Autodesk Inventor part; units mm, degrees
ref_plane "YZ Plane" through (0, 0, 0) normal (1, 0, 0) x (0, 1, 0)
ref_plane "XZ Plane" through (0, 0, 0) normal (0, 1, 0) x (-1, 0, 0)
ref_plane "XY Plane" through (0, 0, 0) normal (0, 0, 1) x (1, 0, 0)
sketch "스케치1" plane through (0, 0, 0) normal (0, 0, 1) x (1, 0, 0)
  line L0 (28.124, 3.5) -> (28.124, -58.5)
  line L1 (-12.7588, 3.5) -> (-12.7588, -58.5)
  line L2 (-12.7588, -58.5) -> (28.124, -58.5)
  line L3 (-12.7588, 3.5) -> (-12.7588, 4.4)
  line L4 (28.124, 4.4) -> (28.124, 3.5)
  line L5 (-12.7588, 4.4) -> (-12.7588, 10)
  line L6 (-12.7588, 10) -> (28.124, 10)
  line L7 (28.124, 10) -> (28.124, 4.4)
  dimension "d16" = 68.5
  dimension "d50" = 40.8828
extrude "돌출2" add sketch "스케치1" along normal blind 4
sketch "스케치4" plane through (0, 0, 4) normal (0, 0, 1) x (1, 0, 0)
  circle A0 centre (7.6826, -9.5) radius 5
  point P0 (0, 0)
sketch "스케치6" plane through (0, 0, 4) normal (0, 0, 1) x (1, 0, 0)
  circle A0 centre (7.6826, -9.5) radius 13 construction
  line L0 (7.6826, -9.5) -> (-1.5098, -0.3076) construction
  line L1 (7.6826, -9.5) -> (20.6826, -9.5) construction
  line L2 (7.6826, -9.5) -> (-1.5098, -18.6924) construction
  line L3 (7.6826, -9.5) -> (20.6826, -9.5) construction
  circle A1 centre (-1.5098, -0.3076) radius 1.6
  circle A2 centre (-1.5098, -18.6924) radius 1.6
  circle A3 centre (7.6826, -9.5) radius 5
  circle A4 centre (16.875, -0.3076) radius 1.6
  line L4 (7.6826, -9.5) -> (16.875, -18.6924) construction
  circle A5 centre (16.875, -18.6924) radius 1.6
  point P0 (0, 0)
  dimension "d51" = 26
  dimension "d52" = 135
  dimension "d53" = 135
  dimension "d54" = 3.2
  dimension "d55" = 3.2
  dimension "d56" = 3.2
  dimension "d57" = 3.2
extrude "돌출4" cut sketch "스케치6" against normal up to surface (4 mm away)
sketch "스케치5" plane through (0, 0, 4) normal (0, 0, 1) x (1, 0, 0)
  line L0 (-12.7588, 10) -> (-12.7588, -58.5)
  line L1 (-12.7588, -58.5) -> (28.124, -58.5)
  line L2 (28.124, -58.5) -> (28.124, 10)
  line L3 (28.124, 10) -> (-12.7588, 10)
  circle A0 centre (-9.7588, -59.5) radius 1.6
  circle A1 centre (25.124, -59.5) radius 1.6
  circle A2 centre (-9.2588, 10.5) radius 1.6
  circle A3 centre (24.624, 10.5) radius 1.6
  line L4 (28.124, 10) -> (28.124, 14)
  line L5 (28.124, -58.5) -> (28.124, 10)
  line L6 (28.124, -58.5) -> (28.124, -62.5)
  point P0 (0, 0)
  dimension "d36" = 3.2
  dimension "d37" = 3.2
  dimension "d38" = 3.2
  dimension "d39" = 3.2
  dimension "d40" = 3
  dimension "d42" = 3.5
  dimension "d44" = 3.5
  dimension "d46" = 3
  dimension "d64" = 4
  dimension "d65" = 3.5
  dimension "d66" = 3.5
  dimension "d67" = 4
  dimension "d68" = 3
  dimension "d69" = 3
extrude "돌출3" cut sketch "스케치5" against normal up to surface (4 mm away) contours A2 L3 | L3 A2 | A0 L1 | L1 A0 | A3 L3 | L3 A3 | A1 L1 | L1 A1
sketch "스케치7" plane through (0, 0, 4) normal (0, 0, 1) x (1, 0, 0)
  line L0 (-12.7588, 10) -> (-12.7588, 14)
  arc A0 (23.1041, 10) -> (26.1439, 10) centre (24.624, 10.5) ccw
  arc A1 (26.373, -58.5) -> (23.875, -58.5) centre (25.124, -59.5) ccw
  arc A2 (-10.7787, 10) -> (-7.7389, 10) centre (-9.2588, 10.5) ccw
  arc A3 (-8.5098, -58.5) -> (-11.0078, -58.5) centre (-9.7588, -59.5) ccw
  circle A4 centre (16.875, -0.3076) radius 1.6
  circle A5 centre (-1.5098, -18.6924) radius 1.6
  circle A6 centre (7.6826, -9.5) radius 5
  circle A7 centre (16.875, -18.6924) radius 1.6
  circle A8 centre (-1.5098, -0.3076) radius 1.6
  line L1 (-12.7588, -58.5) -> (-11.0078, -58.5)
  line L2 (28.124, -58.5) -> (28.124, 10)
  line L3 (28.124, 10) -> (26.1439, 10)
  line L4 (-12.7588, 10) -> (-12.7588, -58.5)
  line L5 (28.124, 10) -> (28.124, 14)
  line L6 (28.124, 14) -> (-12.7588, 14)
  line L7 (28.124, -58.5) -> (28.124, 10)
  line L8 (-12.7588, -58.5) -> (28.124, -58.5)
  line L9 (28.124, -58.5) -> (-12.7588, -58.5)
  line L10 (-12.7588, -58.5) -> (-12.7588, -62.5)
  line L11 (-12.7588, -62.5) -> (28.124, -62.5)
  line L12 (28.124, -62.5) -> (28.124, -58.5)
  line L13 (23.1041, 10) -> (-7.7389, 10)
  line L14 (-10.7787, 10) -> (-12.7588, 10)
  line L15 (-8.5098, -58.5) -> (23.875, -58.5)
  line L16 (26.373, -58.5) -> (28.124, -58.5)
  circle A9 centre (24.624, 10.5) radius 1.6
  arc A10 (-10.7787, 10) -> (-7.7389, 10) centre (-9.2588, 10.5) ccw
  circle A11 centre (-9.2588, 10.5) radius 1.6
  circle A12 centre (25.124, -59.5) radius 1.6
  arc A13 (-8.5098, -58.5) -> (-11.0078, -58.5) centre (-9.7588, -59.5) ccw
  circle A14 centre (-9.7588, -59.5) radius 1.6
  point P0 (0, 0)
  point P1 (26.373, -58.5)
  point P2 (23.875, -58.5)
  point P3 (-7.7389, 10)
  dimension "d60" = 4
  dimension "d61" = 4
extrude "돌출6" add sketch "스케치7" against normal up to surface (4 mm away) contours L0 L6 L5 L3 A9 L13 A11 L14 | L1 A14 L8 A12 L12 L11 L10
fillet "모깎기3" radius 2 4 edges at (28.124, 14, 2) (-12.7588, 14, 2) (-12.7588, -62.5, 2) (28.124, -62.5, 2)
sketch "스케치10" plane through (0, 0, 4) normal (0, 0, 1) x (1, 0, 0)
  line L0 (-3.7588, -53.5) -> (19.124, -53.5)
  line L1 (21.124, -51.5) -> (21.124, -27.5)
  line L2 (19.124, -25.5) -> (-3.7588, -25.5)
  line L3 (-5.7588, -27.5) -> (-5.7588, -51.5)
  circle A0 centre (-9.7588, -59.5) radius 1.6
  line L4 (28.124, -60.5) -> (28.124, 12)
  line L5 (-12.7588, 12) -> (-12.7588, -60.5)
  circle A1 centre (25.124, -59.5) radius 1.6
  circle A2 centre (24.624, 10.5) radius 1.6
  circle A3 centre (-9.2588, 10.5) radius 1.6
  circle A4 centre (16.875, -0.3076) radius 1.6
  circle A5 centre (-1.5098, -18.6924) radius 1.6
  circle A6 centre (7.6826, -9.5) radius 5
  circle A7 centre (16.875, -18.6924) radius 1.6
  circle A8 centre (-1.5098, -0.3076) radius 1.6
  arc A9 (-5.7588, -51.5) -> (-3.7588, -53.5) centre (-3.7588, -51.5) ccw
  arc A10 (19.124, -53.5) -> (21.124, -51.5) centre (19.124, -51.5) ccw
  arc A11 (21.124, -27.5) -> (19.124, -25.5) centre (19.124, -27.5) ccw
  arc A12 (-3.7588, -25.5) -> (-5.7588, -27.5) centre (-3.7588, -27.5) ccw
  arc A13 (26.124, -62.5) -> (28.124, -60.5) centre (26.124, -60.5) ccw
  arc A14 (28.124, 12) -> (26.124, 14) centre (26.124, 12) ccw
  line L6 (26.124, 14) -> (-10.7588, 14)
  arc A15 (-10.7588, 14) -> (-12.7588, 12) centre (-10.7588, 12) ccw
  arc A16 (-12.7588, -60.5) -> (-10.7588, -62.5) centre (-10.7588, -60.5) ccw
  line L7 (-10.7588, -62.5) -> (26.124, -62.5)
  point P0 (0, 0)
  point P1 (-5.7588, -53.5)
  point P2 (21.124, -25.5)
  point P3 (21.124, -53.5)
  point P4 (-5.7588, -25.5)
  dimension "d84" = 16
  dimension "d87" = 7
  dimension "d88" = 7
  dimension "d89" = 2
extrude "돌출7" cut sketch "스케치10" against normal up to surface (4 mm away) contours A9 L3 A12 L2 A11 L1 A10 L0
sketch "스케치11" plane through (0, 0, 4) normal (0, 0, 1) x (1, 0, 0)
  line L0 (-10.7588, 14) -> (26.124, 14)
  line L1 (7.6826, 14) -> (7.6826, -136) construction
  circle A0 centre (7.6826, -79.433) radius 20
  arc A1 (21.124, -27.5) -> (19.124, -25.5) centre (19.124, -27.5) ccw
  line L2 (21.124, -27.5) -> (21.124, -51.5)
  arc A2 (19.124, -53.5) -> (21.124, -51.5) centre (19.124, -51.5) ccw
  line L3 (19.124, -53.5) -> (-3.7588, -53.5)
  arc A3 (-5.7588, -51.5) -> (-3.7588, -53.5) centre (-3.7588, -51.5) ccw
  line L4 (-5.7588, -51.5) -> (-5.7588, -27.5)
  arc A4 (-3.7588, -25.5) -> (-5.7588, -27.5) centre (-3.7588, -27.5) ccw
  line L5 (-3.7588, -25.5) -> (19.124, -25.5)
  circle A5 centre (25.124, -59.5) radius 1.6
  circle A6 centre (-9.7588, -59.5) radius 1.6
  line L6 (28.124, -60.5) -> (28.124, 12)
  line L7 (-12.7588, 12) -> (-12.7588, -60.5)
  circle A7 centre (24.624, 10.5) radius 1.6
  circle A8 centre (-9.2588, 10.5) radius 1.6
  circle A9 centre (16.875, -0.3076) radius 1.6
  circle A10 centre (-1.5098, -18.6924) radius 1.6
  circle A11 centre (7.6826, -9.5) radius 5
  circle A12 centre (16.875, -18.6924) radius 1.6
  circle A13 centre (-1.5098, -0.3076) radius 1.6
  arc A14 (26.124, -62.5) -> (28.124, -60.5) centre (26.124, -60.5) ccw
  arc A15 (28.124, 12) -> (26.124, 14) centre (26.124, 12) ccw
  line L8 (26.124, 14) -> (-10.7588, 14)
  arc A16 (-10.7588, 14) -> (-12.7588, 12) centre (-10.7588, 12) ccw
  arc A17 (-12.7588, -60.5) -> (-10.7588, -62.5) centre (-10.7588, -60.5) ccw
  line L9 (-10.7588, -62.5) -> (26.124, -62.5)
  point P0 (0, 0)
  point P1 (-2.9604, -62.5)
  point P2 (18.3256, -62.5)
  dimension "d90" = 150
  dimension "d91" = 40
  dimension "d92" = 25.933
extrude "돌출8" cut sketch "스케치11" against normal up to surface (4 mm away) contours A0 L9 picked at (6.936, -61.5196)
properties part number "링크2고정부" material "알루미늄 6061"
The listing builds one solid part. Answer for the finished solid, in the listing's coordinates (mm). A direction names the side the tool comes from. Round coordinates to 2 decimals unless told otherwise and drop trailing zeros. Loops run counter-clockwise (first coordinate to the right, second up) from the corner with the lowest first, then second, coordinate; pieces in that order, holes last.
Q1. Which of the six approach directions +Z, -Z, +X, -X, +Y, -Y give full straight-line access (tool end or side, diameter ignored) to faces 1 (the face through (-5.759, -39, 2)), 2 (the face through (28.124, -24, 2))?
Q2. Find the intervals of material crossed by line 1 (X direction, y = 10.5, z = 2.95); line 2 (X direction, y = -44.5, z = 3.5); line 3 (Y direction, x = -10, z = 1.35), in increasing order.
Q3. Section A-A, the plane y = -32 is taken. Determine the outline of the cut face in (x, z), then the cut area to 3 significant figures.
Q4. For a pull along X with two mould halves and no side action, classify faces 3 (the face through (7.84, -59.434, 2.028)), 4 (the face through (7, -24, 0)), 5 (the face through (-12.157, -61.93, 1.972)), 6 (the face through (27.55, -61.9, 1.97)) as released by +X, released by -X, zero draft, split by the parting line, or undercut.
Q5. Given pin 1 Ø3.5 at (x, y) = (-1.51, -0.31) entering from -Z; pin 2 Ø1.2 at (x, z) = (13, 2) entering from -Y, each flat-ended and moving along its own axis, determine where each tip first touches the part or whether it passes through.
Q6. Section C-C, the plane x = 1.5 is taken. Determine the outline of the cut face in (y, z).
Q7. Section D-D, the plane z = 1.2 is taken. Count the separate pieces of the cut face and the enclosed holes in it, then the cut area to 3 significant figures.
Q8. Section B-B, the plane x = 16 is taken. Determine the outline of the cut face in (y, z).
Completed:
1. face 1: +Z, -Z
1. face 2: +Z, -Z, +X, +Y, -Y
2. line 1: x = -12.76 to -10.86, -7.66 to 23.02, 26.22 to 28.12
2. line 2: x = -12.76 to -5.76, 21.12 to 28.12
2. line 3: y = -62.5 to -61.08, -57.92 to 9.08, 11.92 to 14
3. outline: (-12.76, 0) - (-5.76, 0) - (-5.76, 4) - (-12.76, 4) - close; (21.12, 0) - (28.12, 0) - (28.12, 4) - (21.12, 4) - close
3. area: 56.0 mm2
4. face 3: undercut
4. face 4: zero draft
4. face 5: released by -X
4. face 6: released by +X
5. pin 1: stops at z = 0
5. pin 2: stops at y = -60.33
6. outline: (-60.41, 0) - (-53.5, 0) - (-53.5, 4) - (-60.41, 4) - close; (-25.5, 0) - (14, 0) - (14, 4) - (-25.5, 4) - close
7. separate pieces: 1
7. enclosed holes: 10
7. area: 2,190 mm2
8. outline: (-61.24, 0) - (-53.5, 0) - (-53.5, 4) - (-61.24, 4) - close; (-25.5, 0) - (-20.03, 0) - (-20.03, 4) - (-25.5, 4) - close; (-17.35, 0) - (-1.65, 0) - (-1.65, 4) - (-17.35, 4) - close; (1.03, 0) - (14, 0) - (14, 4) - (1.03, 4) - close
